Input: part model. Units: mm. Frame: model coordinates. A direction names the side the tool comes from. Round coordinates to 2 decimals unless told otherwise and drop trailing zeros. Order: outer loops, then holes, each group sorted by start corner. A loop starts at its lowest first (then second) coordinate and runs counter-clockwise, first axis right, second up. Notation, with made-up numbers: (85.25, -38) -> (133.25, -38) arc R22 ccw to (133.25, -21) -> close; hole circle Ø2 at (58, -1). An arc over 180 degrees is marked (long way). Use a Markdown table: item, result.
from build123d import *

# Parameters (mm, degrees)
F0_W     = 20
F0_H     = 50
F1_DEPTH = 10
F2_R     = 1.5
F3_DEPTH = 10.001
F5_DEPTH = 20.001
F7_DEPTH = 10.001


with BuildPart() as f1:
    # F0 (on Top) → F1 (new body)
    with BuildSketch(Plane.XY):
        with Locations((10, 25)):
            Rectangle(F0_W, F0_H)
    extrude(amount=F1_DEPTH)

    # F2 (on face) → F3 (cut, through all)
    with BuildSketch(Plane.XY.offset(10)):
        with Locations((10, 45)):
            Circle(F2_R)
        with Locations((10, 5)):
            Circle(F2_R)
    extrude(amount=-F3_DEPTH, mode=Mode.SUBTRACT)

    # F4 (on face) → F5 (cut, through all)
    with BuildSketch(Plane(origin=(0, 0, 0), x_dir=(0, -1, 0), z_dir=(-1, 0, 0))):
        with BuildLine():
            Line((-42, 0), (-8, 0))
            ThreePointArc((-8, 0), (-9.171573, 2.828427), (-12, 4))
            Line((-12, 4), (-38, 4))
            ThreePointArc((-38, 4), (-40.828427, 2.828427), (-42, 0))
        make_face()
    extrude(amount=-F5_DEPTH, mode=Mode.SUBTRACT)

    # F6 (on face) → F7 (cut, through all)
    with BuildSketch(Plane.XY.offset(10)):
        Polygon((13, 0), (20, 0), (20, 7), align=None)
        Polygon((13, 50), (20, 43), (20, 50), align=None)
    extrude(amount=-F7_DEPTH, mode=Mode.SUBTRACT)


solid = f1.part
1) Draft query along X for faces 1 (the face through (8, 4, 0)), 2 (the face through (0, 25, 6)), 3 (the face through (8.5, 5.07, 5.07)). Return one class per face: released by +X, released by -X, zero draft, split by the parting line, or undercut.
Answer key:
| item | result |
|---|---|
| face 1 | zero draft |
| face 2 | released by -X |
| face 3 | undercut |
2) Cut plane B-B on z = 2.75. Return loops of the section in (x, y), and give its area (3 significant figures).
Answer key:
| item | result |
|---|---|
| outline | (0, 0) -> (13, 0) -> (20, 7) -> (20, 9.1) -> (0, 9.1) -> close; (0, 40.9) -> (20, 40.9) -> (20, 43) -> (13, 50) -> (0, 50) -> close; hole circle Ø3 at (10, 5); hole circle Ø3 at (10, 45) |
| area | 301 mm^2 |
3) Ray query, probe 1 along Y at (x, z) = (10, 6.5); probe 2 along Y at (x, z) = (10, 2); probe 3 along Y at (x, z) = (10, 3.5). Return the intervals inside material, ascending.
Answer key:
| item | result |
|---|---|
| probe 1 | y = 0 to 3.5, 6.5 to 43.5, 46.5 to 50 |
| probe 2 | y = 0 to 3.5, 6.5 to 8.54, 41.46 to 43.5, 46.5 to 50 |
| probe 3 | y = 0 to 3.5, 6.5 to 10.06, 39.94 to 43.5, 46.5 to 50 |
4) Contact query for flat-ended pins moving along their axis: P1, Ø10, axis at x = 12, y = 26.5, coming from the -Z side; P2, Ø1, axis at x = 16, z = 7, coming from the -Y side; P3, Ø1.5, axis at x = 16.5, z = 6, coming from the -Y side. Output: stop coordinate, or through.
Answer key:
| item | result |
|---|---|
| P1 | stops at z = 4 |
| P2 | stops at y = 2.5 |
| P3 | stops at y = 2.75 |
5) Cut plane D-D on z = 8.5. Return loops of the section in (x, y), and give its area (3 significant figures).
Answer key:
| item | result |
|---|---|
| outline | (0, 0) -> (13, 0) -> (20, 7) -> (20, 43) -> (13, 50) -> (0, 50) -> close; hole circle Ø3 at (10, 5); hole circle Ø3 at (10, 45) |
| area | 937 mm^2 |
6) Set-up query: faces 4 (the face through (17, 4, 5)), 5 (the face through (9.86, 40.797, 2.859)). Return all of +Z, -Z, +X, -X, +Y, -Y with unobstructed straight access to the full face (end or side cutting, diameter ignored); none if empty.
Answer key:
| item | result |
|---|---|
| face 4 | +Z, -Z, +X, -Y |
| face 5 | -Z, +X, -X |
7) Cut plane A-A on x = 10. Return loops of the section in (y, z).
Answer key:
| item | result |
|---|---|
| outline | (0, 0) -> (3.5, 0) -> (3.5, 10) -> (0, 10) -> close; (6.5, 0) -> (8, 0) arc R4 cw to (12, 4) -> (38, 4) arc R4 cw to (42, 0) -> (43.5, 0) -> (43.5, 10) -> (6.5, 10) -> close; (46.5, 0) -> (50, 0) -> (50, 10) -> (46.5, 10) -> close |
8) Cut plane C-C on y = 45. Return loops of the section in (x, z).
Answer key:
| item | result |
|---|---|
| outline | (0, 0) -> (8.5, 0) -> (8.5, 10) -> (0, 10) -> close; (11.5, 0) -> (18, 0) -> (18, 10) -> (11.5, 10) -> close |
